```python
from build123d import *

# Parameters (mm, degrees)
F0_R     = 101.6
F0_R_2   = 4.7625
F1_DEPTH = 12.7
F1_TAPER = 1.5
F0_R_3   = 111.125
F2_DEPTH = 5.08


with BuildPart() as f1:
    # F0 (on Front) → F1 (new body)
    with BuildSketch(Plane.XZ):
        Circle(F0_R)
        Circle(F0_R_2, mode=Mode.SUBTRACT)
    extrude(amount=-F1_DEPTH, taper=F1_TAPER)

    # F0 (on Front) → F2 (join)
    with BuildSketch(Plane.XZ):
        Circle(F0_R_3)
        Circle(F0_R, mode=Mode.SUBTRACT)
        Circle(F0_R)
        Circle(F0_R_2, mode=Mode.SUBTRACT)
    extrude(amount=F2_DEPTH)


solid = f1.part
```
Check sheet for the modelled part. Datum: model origin and axes. Units: mm. A direction names the side the tool comes from. Give positions to 0.01 mm unless a question says otherwise; leave off trailing zeros. Write each loop counter-clockwise with the first axis right and the second up, starting at its lowest first coordinate (ties: lowest second). Pieces come first, ordered by that corner, then holes. Notation, with made-up numbers: (7.25, 23) - (23.25, 23) arc R31 ccw to (23.25, 58) - close; hole circle Ø3 at (-7.5, -20.75). An arc over 180 degrees is marked (long way). Answer as a JSON object with one key per item and string values. Group by question number.
1) Sectioned sample at B-B (y = 4). Record the cut outline in (x, z), then the cut area to 3 significant figures.
2) Depth check by flat-ended pin: P1, Ø1, axis at y = -1.5, z = 76, coming from the +X side; P2, Ø4, axis at y = 1.5, z = -53.5, coming from the +X side; P3, Ø1, axis at y = 9.5, z = -1, coming from the +X side. Enter the tip coordinate at first touch or a pass-through.
3) Release check for a two-part mould opening along Z. For faces 1 (the face through (-2, -5.08, -23)), 2 (the face through (-14.47, -2.5, 110.18)), 3 (the face through (-3.78, -2.5, -2.9)) record: pulls with the +Z half, pulls with the -Z half, needs draft (parallel to the pull), parting line crosses it, or undercut.
4) Sectioned sample at A-A (x = 0). Record the cut outline in (y, z) (1 decimal), then the cut area to 3 significant figures.
5) Access from +Z, -Z, +X, -X, +Y, -Y to the whole of each face (thin tool, end or side, straight path). Record for faces 4 (the face through (-0.64, 6.44, -4.89)), 5 (the face through (21, 12.7, 1)).
6) Thickness scan on probe 1 along Z at (x, y) = (0, -3.7) (1 decimal); probe 2 along X at (y, z) = (12, 4); probe 3 along X at (y, z) = (3, -55). Record the ranges inside material, lowest first. Write a range as from..to.
Geometry results:
{
 "1": {"outline": "circle Ø202.99 at (0, 0); hole circle Ø9.73 at (0, 0)", "area": "32,300 mm^2"},
 "2": {"P1": "stops at x = 81.54", "P2": "stops at x = 98.11", "P3": "stops at x = 101.36"},
 "3": {"face 1": "needs draft", "face 2": "parting line crosses it", "face 3": "undercut"},
 "4": {"outline": "(-5.1, -111.1) - (0, -111.1) - (0, -101.6) - (12.7, -101.3) - (12.7, -5.1) - (0, -4.8) - (-5.1, -4.8) - close; (-5.1, 4.8) - (0, 4.8) - (12.7, 5.1) - (12.7, 101.3) - (0, 101.6) - (0, 111.1) - (-5.1, 111.1) - close", "area": "3,530 mm^2"},
 "5": {"face 4": "+Y", "face 5": "+Z, -Z, +X, -X, +Y"},
 "6": {"probe 1": "z = -111.1..-4.8, 4.8..111.1", "probe 2": "x = -101.21..-3.13, 3.13..101.21", "probe 3": "x = -85.33..85.33"}
}
